CAD build for the part. Positions are in the model's coordinates, mm. A direction names the side the tool comes from. Round coordinates to 2 decimals unless told otherwise and drop trailing zeros. Put each result on its own line as item: value. Start each with the question number.
from build123d import *

# Parameters (mm, degrees)
SKETCH_1_W              = 23.5
SKETCH_1_H              = 12
EXTRUDE_1_DEPTH         = 495.5
HOLE_WIZARD_M6_1_D      = 5
HOLE_WIZARD_M6_1_DEPTH  = 19
HOLE_WIZARD_M6_1_TIP    = 1.502151548
HOLE_WIZARD_M6_2_D      = 5
HOLE_WIZARD_M6_2_DEPTH  = 19
HOLE_WIZARD_M6_2_TIP    = 1.502151548
HOLE_WIZARD_M6_3_D      = 5
HOLE_WIZARD_M6_3_DEPTH  = 19
HOLE_WIZARD_M6_3_TIP    = 1.502151548
HOLE_WIZARD_12_0_12_1_D = 12
HOLE_WIZARD_M4_1_D      = 3.3
HOLE_WIZARD_M4_1_DEPTH  = 11.5
HOLE_WIZARD_M4_1_TIP    = 0.991420021


with BuildPart() as part:
    # 草图1 → 凸台-拉伸1 (new, symmetric)
    with BuildSketch(Plane(origin=(0, 0, 0), x_dir=(0, 0, -1), z_dir=(1, 0, 0))):
        Polygon((-15, 15), (-11.5, 15), (-11.5, 13.5), (-11, 13.5), (-11, 12), (-9.5, 12), (-9.5, 15), (-8, 15), (-8, 12.5), (-5, 12.5), (-5, 15), (5, 15), (5, 12.5), (8, 12.5), (8, 15), (9.5, 15), (9.5, 12), (11, 12), (11, 13.5), (11.5, 13.5), (11.5, 15), (15, 15), (15, 8), (12.5, 8), (12.5, 5), (15, 5), (15, -5), (12.5, -5), (12.5, -8), (15, -8), (15, -15), (11.5, -15), (11.5, -13.5), (11, -13.5), (11, -12), (9.5, -12), (9.5, -15), (8, -15), (8, -12.5), (5, -12.5), (5, -15), (-5, -15), (-5, -12.5), (-8, -12.5), (-8, -15), (-9.5, -15), (-9.5, -12), (-11, -12), (-11, -13.5), (-11.5, -13.5), (-11.5, -15), (-15, -15), align=None)
        with BuildLine():
            Line((12, -10.5), (12, -8.5))
            ThreePointArc((12, -8.5), (11.853553391, -8.146446609), (11.5, -8))
            Line((11.5, -8), (-11.5, -8))
            ThreePointArc((-11.5, -8), (-11.853553391, -8.146446609), (-12, -8.5))
            Line((-12, -8.5), (-12, -10.5))
            ThreePointArc((-12, -10.5), (-11.853553391, -10.853553391), (-11.5, -11))
            Line((-11.5, -11), (11.5, -11))
            ThreePointArc((11.5, -11), (11.853553391, -10.853553391), (12, -10.5))
        make_face(mode=Mode.SUBTRACT)
        with BuildLine():
            Line((-11.5, 11), (11.5, 11))
            ThreePointArc((11.5, 11), (11.853553391, 10.853553391), (12, 10.5))
            Line((12, 10.5), (12, 8.5))
            ThreePointArc((12, 8.5), (11.853553391, 8.146446609), (11.5, 8))
            Line((11.5, 8), (-11.5, 8))
            ThreePointArc((-11.5, 8), (-11.853553391, 8.146446609), (-12, 8.5))
            Line((-12, 8.5), (-12, 10.5))
            ThreePointArc((-12, 10.5), (-11.853553391, 10.853553391), (-11.5, 11))
        make_face(mode=Mode.SUBTRACT)
        Rectangle(SKETCH_1_W, SKETCH_1_H, mode=Mode.SUBTRACT)
    extrude(amount=EXTRUDE_1_DEPTH, both=True)

    # M6 螺纹孔1
    with Locations(Plane(origin=(0, -15, 0), x_dir=(-1, 0, 0), z_dir=(0, -1, 0))):
        with Locations((-445.5, 0), (-430.5, 0), (230.5, 0), (245.5, 0), (460.5, 0), (475.5, 0)):
            Hole(HOLE_WIZARD_M6_1_D / 2, depth=HOLE_WIZARD_M6_1_DEPTH)
            with Locations((0, 0, -(HOLE_WIZARD_M6_1_DEPTH + HOLE_WIZARD_M6_1_TIP / 2))):  # 118° drill point
                Cone(0, HOLE_WIZARD_M6_1_D / 2, HOLE_WIZARD_M6_1_TIP, mode=Mode.SUBTRACT)

    # M6 螺纹孔2
    with Locations(Plane(origin=(0, 0, -15), x_dir=(-1, 0, 0), z_dir=(0, 0, -1))):
        with Locations((-445.5, 0), (-430.5, 0), (-370.5, 0), (-266.5, 0), (-394.5, 0)):
            Hole(HOLE_WIZARD_M6_2_D / 2, depth=HOLE_WIZARD_M6_2_DEPTH)
            with Locations((0, 0, -(HOLE_WIZARD_M6_2_DEPTH + HOLE_WIZARD_M6_2_TIP / 2))):  # 118° drill point
                Cone(0, HOLE_WIZARD_M6_2_D / 2, HOLE_WIZARD_M6_2_TIP, mode=Mode.SUBTRACT)

    # M6 螺纹孔3
    with Locations(Plane(origin=(0, 15, 0), x_dir=(1, 0, 0), z_dir=(0, 1, 0))):
        with Locations((133, 0), (118, 0), (-460.5, 0), (-475.5, 0), (-167, 0)):
            Hole(HOLE_WIZARD_M6_3_D / 2, depth=HOLE_WIZARD_M6_3_DEPTH)
            with Locations((0, 0, -(HOLE_WIZARD_M6_3_DEPTH + HOLE_WIZARD_M6_3_TIP / 2))):  # 118° drill point
                Cone(0, HOLE_WIZARD_M6_3_D / 2, HOLE_WIZARD_M6_3_TIP, mode=Mode.SUBTRACT)

    # Ø12.0 (12) 直径孔1 (through all)
    with Locations(Plane(origin=(0, -15, 0), x_dir=(-1, 0, 0), z_dir=(0, -1, 0))):
        with Locations((-168, 0), (405.5, 0)):
            Hole(HOLE_WIZARD_12_0_12_1_D / 2)

    # M4 螺纹孔1
    with Locations(Plane(origin=(0, 0, -15), x_dir=(-1, 0, 0), z_dir=(0, 0, -1))):
        with Locations((-341, 0), (-296, 0), (-236, 0), (-191, 0)):
            Hole(HOLE_WIZARD_M4_1_D / 2, depth=HOLE_WIZARD_M4_1_DEPTH)
            with Locations((0, 0, -(HOLE_WIZARD_M4_1_DEPTH + HOLE_WIZARD_M4_1_TIP / 2))):  # 118° drill point
                Cone(0, HOLE_WIZARD_M4_1_D / 2, HOLE_WIZARD_M4_1_TIP, mode=Mode.SUBTRACT)


solid = part.part
(1) Drill centre lines: line 1 along Y through (x, z) = (-174, 1); line 2 along Y through (x, z) = (445.5, -12.8); line 3 along Z through (x, y) = (339, -1.75). Where is each one in solid material? Low to high.
(2) Mould opens along Y. For faces 3 (the flat face through (7, -6, 0)), 4 (the flat face through (-495.5, 7, 0)) say: +Y half, -Y half, draft (parallel to the pull), parting line (faces both ways), or undercut.
(3) Flat gauge pins, fed straight in: pin 1 Ø4 at (x, z) = (-245.5, 0) entering from -Y; pin 2 Ø0.9 at (x, z) = (-53, 6) entering from -Y. Where does each tip first touch, or does it go through?
(4) Cut at A-A on x = -17. Count the separate pieces of the cut face and the enclosed holes in it, and give its area (3 significant figures).
(5) Tool access for faces 1 (the flat face through (7, 6, 0)), 2 (the flat face through (495.5, 7, 0)): list every direction of +Z, -Z, +X, -X, +Y, -Y with a clear straight run to the whole face (end or side of a thin tool).
Taken from the geometry:
1. line 1: -15 to -11, -8 to -6, 6 to 8, 11 to 15
1. line 2: -15 to -8, -5 to -2.5, 2.5 to 5, 8 to 15
1. line 3: -15 to -11.75, 11.75 to 15
2. face 3: undercut
2. face 4: draft
3. pin 1: y = 6
3. pin 2: y = -12.5
4. separate pieces: 1
4. enclosed holes: 3
4. area: 408 mm2
5. face 1: +X, -X
5. face 2: +Z, -Z, +X, +Y, -Y
